```python
from build123d import *

# Parameters (mm, degrees)
CROQUIS1_W              = 55
CROQUIS1_H              = 40
CROQUIS1_W_2            = 5
CROQUIS1_H_2            = 25
SALIENTE_EXTRUIR1_DEPTH = 5.5


with BuildPart() as part:
    # Croquis1 → Saliente-Extruir1 (new body)
    with BuildSketch(Plane.XY):
        Polygon((-71.983561291, 36.108229285), (-71.983561291, 9.858229285), (-66.483561291, 9.858229285), (-66.483561291, -10.141770715), (-71.983561291, -10.141770715), (-71.983561291, -41.891770715), (36.016438709, -41.891770715), (36.016438709, -36.391770715), (144.016438709, -36.391770715), (144.016438709, -41.891770715), (252.016438709, -41.891770715), (252.016438709, -36.391770715), (360.016438709, -36.391770715), (360.016438709, -41.891770715), (468.016438709, -41.891770715), (468.016438709, 88.608229285), (438.016438709, 88.608229285), (438.016438709, 83.108229285), (373.516438709, 83.108229285), (373.516438709, 88.608229285), (343.516438709, 88.608229285), (343.516438709, 73.608229285), (338.016438709, 73.608229285), (338.016438709, 53.608229285), (343.516438709, 53.608229285), (343.516438709, 36.108229285), (338.016438709, 36.108229285), (256.016438709, 36.108229285), (256.016438709, 41.608229285), (174.016438709, 41.608229285), (174.016438709, 36.108229285), (92.016438709, 36.108229285), (92.016438709, 41.608229285), (10.016438709, 41.608229285), (10.016438709, 36.108229285), align=None)
        with Locations((403.016438709, 58.608229285)):
            Rectangle(CROQUIS1_W, CROQUIS1_H, mode=Mode.SUBTRACT)
        with Locations((367.016438709, 0)):
            Rectangle(CROQUIS1_W_2, CROQUIS1_H_2, mode=Mode.SUBTRACT)
    extrude(amount=SALIENTE_EXTRUIR1_DEPTH)


solid = part.part
```
The listing builds one solid part. Answer for the finished solid, in the listing's coordinates (mm). Round coordinates to 2 decimals unless told otherwise and drop trailing zeros. Write each loop counter-clockwise with the first axis right and the second up, starting at its lowest first coordinate (ties: lowest second). Pieces come first, ordered by that corner, then holes. Notation, with made-up numbers: (2.25, 9.5) -> (10.25, 9.5) arc R27 ccw to (10.25, 47.5) -> close; hole circle Ø2 at (-25, 6.25). An arc over 180 degrees is marked (long way). Use CSV: the item, a comma, the result in double quotes. Start each with the question number.
(1) Section C-C on z = 1.65 is taken. Count the separate pieces of the cut face and the enclosed holes in it, then the cut area to 3 significant figures.
(2) Section A-A on x = 410.5 is taken. Give the vertices of the cut face in (y, z), then the cut area to 4 significant figures.
(3) Section B-B on y = -1 is taken. Give the vertices of the cut face in (x, z), then the cut area to 3 significant figures.
(4) Section D-D on x = 206 is taken. Give the vertices of the cut face in (y, z), then the cut area to 3 significant figures.
(5) Consider L1, parallel to X at y = -10, z = 2.15; L2, parallel to X at y = 46.5, z = 1.5; L3, parallel to Y at x = 342.5, z = 3.5. Determine where each line is inside the solid, lowest interval first. Write a range as from..to.
(6) Each of these flat-tipped pins is pushed along its axis until it touches: pin 1 (1.6 mm diameter, centred on y = 80, z = 2.5, fed in from -X); pin 2 (3 mm diameter, centred on y = 2.5, z = 3.5, fed in from -X); pin 3 (1.6 mm diameter, centred on x = 341.5, z = 3, fed in from +Y). Where does it stop, or does it pass through?
A:
1,separate pieces,"1"
1,enclosed holes,"2"
1,area,"45,700 mm²"
2,outline,"(-41.89, 0) -> (38.61, 0) -> (38.61, 5.5) -> (-41.89, 5.5) -> close; (78.61, 0) -> (83.11, 0) -> (83.11, 5.5) -> (78.61, 5.5) -> close"
2,area,"467.5 mm²"
3,outline,"(-66.48, 0) -> (364.52, 0) -> (364.52, 5.5) -> (-66.48, 5.5) -> close; (369.52, 0) -> (468.02, 0) -> (468.02, 5.5) -> (369.52, 5.5) -> close"
3,area,"2,910 mm²"
4,outline,"(-41.89, 0) -> (41.61, 0) -> (41.61, 5.5) -> (-41.89, 5.5) -> close"
4,area,"459 mm²"
5,L1,"x = -66.48..364.52, 369.52..468.02"
5,L2,"x = 343.52..375.52, 430.52..468.02"
5,L3,"y = -36.39..36.11, 53.61..73.61"
6,pin 1,"stops at x = 343.52"
6,pin 2,"stops at x = -66.48"
6,pin 3,"stops at y = 73.61"
